CAD build for the part. Positions are in the model's coordinates, mm. A direction names the side the tool comes from. Give positions to 0.01 mm unless a question says otherwise; leave off trailing zeros. Order: outer loops, then holes, each group sorted by start corner. A loop starts at its lowest first (then second) coordinate and runs counter-clockwise, first axis right, second up. Notation, with made-up numbers: M 35.5,37.5 L 92.5,37.5 A18 cw 92.5,68.5 Z; hole C -31,-30 d7. An arc over 180 degrees is marked long. Put each result on its own line as item: value. Start each with the question number.
1) Cut at A-A (y = 26.5). Write the cut outline in (x, z).
2) Tool access for faces 1 (the face through (13.043, 29, 0)), 2 (the face through (0, 6.35, -45)), 3 (the face through (0, 19.05, -22)): list every direction of +Z, -Z, +X, -X, +Y, -Y with a clear straight run to the whole face (end or side of a thin tool).
3) Pin check, flat tips, straight feed: pin 1 (21 mm diameter, centred on x = -6, y = 25.5, fed in from -Z); pin 2 (23 mm diameter, centred on y = 44.45, z = 0, fed in from -X); pin 3 (5.5 mm diameter, centred on y = 44.45, z = -22.225, fed in from -X); pin 4 (10 mm diameter, centred on x = -5.5, y = 13, fed in from +Z). Stop position of each tip, or through.
4) Cut at C-C (y = 44.45). Give the number of separate pieces and of enclosed holes in the cut face, and give its area (3 significant figures).
5) Cut at D-D (x = -4). Write the cut outline in (y, z).
6) Drill centre lines: line 1 (Z direction, x = -16.75, y = 44.45); line 2 (Y direction, x = 16.25, z = 0); line 3 (X direction, y = 39.5, z = 21). Where is each one in solid material? Low to high. Write a range as [from, to].
7) Two-plate mould, pull along Z, no slides. Class faces 4 (the face through (-14, 29, 25.4)), 5 (the face through (-17.099, 42.859, 23.684)), 6 (the face through (0, 0, -1)): released by +Z, released by -Z, zero draft, split by the parting line, or undercut.
8) Cut at B-B (z = 0). Write the cut outline in (x, y).
```python
from build123d import *

# Parameters (mm, degrees)
BOSS_EXTRUDE1_DEPTH     = 25.4
CUT_EXTRUDE1_DEPTH      = 81.304376648
CUT_EXTRUDE1_DEPTH_BACK = 81.304376648
SKETCH2_R               = 14.2875
SKETCH2_R_2             = 2.159
SKETCH3_W               = 42.0878
SKETCH3_H               = 127
BOSS_EXTRUDE2_DEPTH     = 6.35
SKETCH4_W               = 26.0858
SKETCH4_H               = 12.7
BOSS_EXTRUDE3_DEPTH     = 6.35


with BuildPart() as part:
    # Sketch1 → Boss-Extrude1 (new, symmetric)
    with BuildSketch(Plane.XY):
        Polygon((-21.0439, 0), (21.0439, 0), (21.0439, 63.5), (13.0429, 63.5), (13.0429, 6.35), (-13.0429, 6.35), (-13.0429, 63.5), (-21.0439, 63.5), align=None)
    extrude(amount=BOSS_EXTRUDE1_DEPTH, both=True)

    # Sketch2 → Cut-Extrude1 (cut, two sides: drawn at the far end of the back side and taken through both)
    with BuildSketch(Plane(origin=(21.0439, 0, 0), x_dir=(0, 0, -1), z_dir=(1, 0, 0)).offset(-CUT_EXTRUDE1_DEPTH_BACK)):
        with Locations(Location((0, 44.45, 0), (0, 0, 90))):
            Circle(SKETCH2_R)
        with Locations(Location((22.225, 44.45, 0), (0, 0, 90))):
            Circle(SKETCH2_R_2)
        with Locations(Location((-22.225, 44.45, 0), (0, 0, 90))):
            Circle(SKETCH2_R_2)
    extrude(amount=CUT_EXTRUDE1_DEPTH + CUT_EXTRUDE1_DEPTH_BACK, mode=Mode.SUBTRACT)

    # Sketch3 → Boss-Extrude2 (add)
    with BuildSketch(Plane(origin=(0, 0, 0), x_dir=(-1, 0, 0), z_dir=(0, -1, 0))):
        Rectangle(SKETCH3_W, SKETCH3_H)
    extrude(amount=-BOSS_EXTRUDE2_DEPTH)

    # Sketch4 → Boss-Extrude3 (add)
    with BuildSketch(Plane(origin=(0, 0, -25.4), x_dir=(-1, 0, 0), z_dir=(0, 0, -1))):
        with Locations((0, 12.7)):
            Rectangle(SKETCH4_W, SKETCH4_H)
    boss_extrude3 = extrude(amount=-BOSS_EXTRUDE3_DEPTH)

    # Mirror1: Boss-Extrude3 across plane
    add(boss_extrude3.mirror(Plane.XY))


solid = part.part
```
Solution:
1. outline: M -21.04,-25.4 L -13.04,-25.4 L -13.04,25.4 L -21.04,25.4 Z; M 13.04,-25.4 L 21.04,-25.4 L 21.04,25.4 L 13.04,25.4 Z
2. face 1: +Y
2. face 2: -Z, +X, -X, +Y
2. face 3: +Z, -Z, +Y
3. pin 1: z = -25.4
3. pin 2: through
3. pin 3: x = -21.04
3. pin 4: z = 25.4
4. separate pieces: 8
4. enclosed holes: 0
4. area: 217 mm²
5. outline: M 0,-63.5 L 6.35,-63.5 L 6.35,-25.4 L 19.05,-25.4 L 19.05,-19.05 L 6.35,-19.05 L 6.35,19.05 L 19.05,19.05 L 19.05,25.4 L 6.35,25.4 L 6.35,63.5 L 0,63.5 Z
6. line 1: [-25.4, -24.38], [-20.07, -14.29], [14.29, 20.07], [24.38, 25.4]
6. line 2: [0, 30.16], [58.74, 63.5]
6. line 3: [-21.04, -13.04], [13.04, 21.04]
7. face 4: released by +Z
7. face 5: undercut
7. face 6: zero draft
8. outline: M -21.04,0 L 21.04,0 L 21.04,30.16 L 13.04,30.16 L 13.04,6.35 L -13.04,6.35 L -13.04,30.16 L -21.04,30.16 Z; M -21.04,58.74 L -13.04,58.74 L -13.04,63.5 L -21.04,63.5 Z; M 13.04,58.74 L 21.04,58.74 L 21.04,63.5 L 13.04,63.5 Z
